Read the model definition and answer for the solid it produces. Units are mm, in the model's axes. Face numbers are marked on the shaded views. A direction names the side the tool comes from. Round coordinates to 2 decimals unless told otherwise and drop trailing zeros. Write each loop counter-clockwise with the first axis right and the second up, starting at its lowest first coordinate (ties: lowest second). Pieces come first, ordered by that corner, then holes. Notation, with made-up numbers: (71, -13) -> (80, -13) arc R37 cw to (80, 25) -> close; hole circle Ø6 at (30, -2). An arc over 180 degrees is marked (long way). Return JSON: item names as keys, results as strings. Group by question number.
(1) A cutting plane is placed at B-B on y = 7.25. Give the vertices of the cut face in (x, z), then the cut area to 4 significant figures.
(2) Straight lines are drawn through the part: line 1 (X direction, y = 2.25, z = -26); line 2 (Y direction, x = 3.5, z = -27.5). For each, find the intervals that lie inside material, in ascending order.
(3) A cutting plane is placed at A-A on z = -17.5. Give the vertices of the cut face in (x, y).
(4) A cutting plane is placed at C-C on z = -27.5. Give the vertices of the cut face in (x, y).
(5) Given pin 1 (2 mm diameter, centred on x = -125.5, y = 6.5, fed in from +Z); pin 2 (12 mm diameter, centred on y = 15.5, z = -16.5, fed in from -X); pin 3 (5 mm diameter, centred on y = 20.5, z = -4.5, fed in from +X); pin 4 (7.5 mm diameter, centred on x = -225.5, z = -23.5, fed in from -Y), each flat-ended and moving along its own axis, determine where each tip first touches the part or whether it passes through.
(6) For the marked faces 1, 2 and 3, determine the directions among +Z, -Z, +X, -X, +Y, -Y from which every point of the face is accessible in a straight line to the end or side of a thin tool.
Autodesk Inventor part; units mm, degrees
ref_plane "YZ Plane" through (0, 0, 0) normal (1, 0, 0) x (0, 1, 0)
ref_plane "XZ Plane" through (0, 0, 0) normal (0, 1, 0) x (-1, 0, 0)
ref_plane "XY Plane" through (0, 0, 0) normal (0, 0, 1) x (1, 0, 0)
sketch "Sketch1" plane through (0, 0, 0) normal (0, 1, 0) x (-1, 0, 0)
  line L0 (0, 0) -> (215, 0)
  line L1 (215, 0) -> (215, -35)
  line L2 (215, -35) -> (0, -35)
  line L3 (0, -35) -> (0, 0)
  dimension "d0" = 215
  dimension "d1" = 35
extrude "Extrusion1" add sketch "Sketch1" along normal blind 27
sketch "Sketch2" plane through (0, 27, 0) normal (0, 1, 0) x (1, 0, 0)
  line L0 (0, 0) -> (15, 0)
  line L1 (15, 0) -> (15, 35)
  line L2 (15, 35) -> (0, 35)
  line L3 (0, 35) -> (0, 0)
  line L4 (-215, 35) -> (-215, 0)
  line L5 (-215, 0) -> (-230, 0)
  line L6 (-230, 0) -> (-230, 35)
  line L7 (-230, 35) -> (-215, 35)
  line L8 (-215, 35) -> (-215, 0)
  dimension "d4" = 15
  dimension "d5" = 35
  dimension "d6" = 15
  dimension "d7" = 35
extrude "Extrusion2" add sketch "Sketch2" against normal blind 1
sketch "Sketch3" plane through (0, 27, 0) normal (0, 1, 0) x (1, 0, 0)
  line L0 (15, 13.5) -> (8, 13.5)
  line L1 (4, 17.5) -> (4, 17.5)
  line L2 (8, 21.5) -> (15, 21.5)
  line L3 (15, 21.5) -> (15, 13.5)
  line L4 (15, 35) -> (-230, 35)
  line L5 (15, 0) -> (15, 35)
  line L6 (-230, 13.5) -> (-223, 13.5)
  line L7 (-219, 17.5) -> (-219, 17.5)
  line L8 (-223, 21.5) -> (-230, 21.5)
  line L9 (-230, 21.5) -> (-230, 13.5)
  line L10 (15, 0) -> (-230, 0)
  arc A0 (-223, 13.5) -> (-219, 17.5) centre (-223, 17.5) ccw
  arc A1 (-219, 17.5) -> (-223, 21.5) centre (-223, 17.5) ccw
  line L11 (-230, 0) -> (-230, 35)
  arc A2 (4, 17.5) -> (8, 13.5) centre (8, 17.5) ccw
  arc A3 (8, 21.5) -> (4, 17.5) centre (8, 17.5) ccw
  point P0 (0, 0)
  point P1 (4, 21.5)
  point P2 (4, 13.5)
  point P3 (-219, 21.5)
  point P4 (-219, 13.5)
  dimension "d10" = 11
  dimension "d11" = 8
  dimension "d12" = 13.5
  dimension "d13" = 0
  dimension "d14" = 11
  dimension "d15" = 8
  dimension "d16" = 13.5
  dimension "d17" = 4
  dimension "d18" = 4
  dimension "d19" = 0
  dimension "d20" = 4
extrude "Extrusion3" cut sketch "Sketch3" against normal blind 1 contours L0 A2 A3 L2 L3 | L9 L8 A1 A0 L6
properties part number "Balastro"
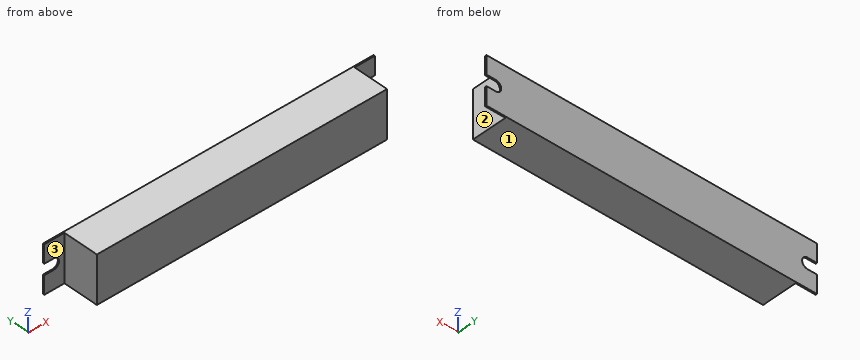
Checks:
{
 "1": {"outline": "(-215, -35) -> (0, -35) -> (0, 0) -> (-215, 0) -> close", "area": "7,525 mm^2"},
 "2": {"line 1": "x = -215 to 0", "line 2": "y = 26 to 27"},
 "3": {"outline": "(-219, 26) -> (-215, 26) -> (-215, 0) -> (0, 0) -> (0, 26) -> (4, 26) -> (4, 27) -> (-219, 27) -> close"},
 "4": {"outline": "(-230, 26) -> (-215, 26) -> (-215, 0) -> (0, 0) -> (0, 26) -> (15, 26) -> (15, 27) -> (-230, 27) -> close"},
 "5": {"pin 1": "stops at z = 0", "pin 2": "stops at x = -215", "pin 3": "stops at x = 0", "pin 4": "stops at y = 26"},
 "6": {"face 1": "-Z, +X, -X, +Y, -Y", "face 2": "+Z, -Z, +X, -Y", "face 3": "+Z, -Z, -X, -Y"}
}
